Geometry: final body of the model. Coordinates: model frame, mm. A direction names the side the tool comes from. Give positions to 0.01 mm unless a question says otherwise; leave off trailing zeros. Loops run counter-clockwise (first coordinate to the right, second up) from the corner with the lowest first, then second, coordinate; pieces in that order, holes last.
from build123d import *

# Parameters (mm, degrees)
F0_W     = 1092.2
F0_H     = 744.5375
F0_W_2   = 920.75
F0_H_2   = 514.35
F1_DEPTH = 127
F2_W     = 1066.8
F2_H     = 25.4
F3_DEPTH = 25.4
F4_SIZE  = 9.525
F5_R     = 12.7
F6_DEPTH = 1066.8
F8_DEPTH = 6.35


with BuildPart() as f1:
    # F0 (on Top) → F1 (new body)
    with BuildSketch(Plane.XY):
        with Locations((546.1, 372.26875)):
            Rectangle(F0_W, F0_H)
        with Locations((527.05, 382.5875)):
            Rectangle(F0_W_2, F0_H_2, mode=Mode.SUBTRACT)
    extrude(amount=F1_DEPTH)

    # F2 (on face) → F3 (join)
    with BuildSketch(Plane.XY.offset(127)):
        with Locations((546.1, 31.75)):
            Rectangle(F2_W, F2_H)
        with Locations((546.1, 708.025)):
            Rectangle(F2_W, F2_H)
    extrude(amount=F3_DEPTH)

    # F4
    f4_edges = [f1.edges().sort_by_distance(p)[0] for p in [
        (546.1, 19.05, 152.4),
        (546.1, 44.45, 152.4),
        (546.1, 720.725, 152.4),
        (546.1, 695.325, 152.4),
    ]]
    chamfer(f4_edges, length=F4_SIZE)

    # F5 (on face) → F6 (join)
    with BuildSketch(Plane(origin=(12.7, 0, 0), x_dir=(0, -1, 0), z_dir=(-1, 0, 0))):
        with Locations((-708.025, 158.75)):
            Circle(F5_R)
        with BuildLine():
            Line((-34.925, 152.4), (-39.001326, 148.323674))
            ThreePointArc((-39.001326, 148.323674), (-31.75, 146.05), (-24.498674, 148.323674))
            Line((-24.498674, 148.323674), (-28.575, 152.4))
            Line((-28.575, 152.4), (-34.925, 152.4))
        make_face()
        with BuildLine():
            ThreePointArc((-24.498674, 148.323674), (-20.494294, 152.867902), (-19.05, 158.75))
            ThreePointArc((-19.05, 158.75), (-37.632098, 170.005706), (-39.001326, 148.323674))
            Line((-39.001326, 148.323674), (-34.925, 152.4))
            Line((-34.925, 152.4), (-28.575, 152.4))
            Line((-28.575, 152.4), (-24.498674, 148.323674))
        make_face()
    extrude(amount=-F6_DEPTH)

    # F7 (on face) → F8 (join)
    with BuildSketch(Plane.XY.offset(127)):
        Polygon((0, 0), (31.75, 0), (31.75, 19.05), (12.7, 19.05), (12.7, 44.45), (31.75, 44.45), (31.75, 133.35), (0, 133.35), align=None)
        Polygon((0, 744.5375), (0, 611.1875), (31.75, 611.1875), (31.75, 695.325), (12.7, 695.325), (12.7, 720.725), (31.75, 720.725), (31.75, 744.5375), align=None)
        Polygon((1060.45, 611.1875), (1092.2, 611.1875), (1092.2, 744.5375), (1060.45, 744.5375), (1060.45, 720.725), (1079.5, 720.725), (1079.5, 695.325), (1060.45, 695.325), align=None)
        Polygon((1060.45, 0), (1092.2, 0), (1092.2, 133.35), (1060.45, 133.35), (1060.45, 44.45), (1079.5, 44.45), (1079.5, 19.05), (1060.45, 19.05), align=None)
    extrude(amount=F8_DEPTH)


solid = f1.part
Item 1: Section query C-C on y = 560. Return loops of the section in (x, z) (3 decimals), plus the area to 3 significant figures.
Values follow:
outline: (0, 0) - (66.675, 0) - (66.675, 127) - (0, 127) - close; (987.425, 0) - (1092.2, 0) - (1092.2, 127) - (987.425, 127) - close
area: 21,800 mm2
Item 2: Set-up query: faces 1 (the face through (1079.5, 32, 152)), 2 (the face through (66.675, 379, 63)), 3 (the face through (12.7, 708, 153)). Return all of +Z, -Z, +X, -X, +Y, -Y with unobstructed straight access to the full face (end or side cutting, diameter ignored); none if empty.
Values follow:
face 1: +Z, +X, +Y, -Y
face 2: +Z, -Z
face 3: +Z, -X, +Y, -Y
Item 3: Section query A-A on z = 15.5. Return loops of the section in (x, y) (1 decimal).
Values follow:
outline: (0, 0) - (1092.2, 0) - (1092.2, 744.5) - (0, 744.5) - close; hole (66.7, 125.4) - (987.4, 125.4) - (987.4, 639.8) - (66.7, 639.8) - close
Item 4: Pin query (flat end, axial travel): pin 1 (8 mm diameter, centred on x = 785, z = 136, fed in from -Y); pin 2 (12.5 mm diameter, centred on y = 710, z = 158.5, fed in from -X); pin 3 (5 mm diameter, centred on x = 686.5, z = 138, fed in from +Y) (3 decimals). Return the tip coordinate at first contact, or that it passes through.
Values follow:
pin 1: stops at y = 19.05
pin 2: stops at x = 12.7
pin 3: stops at y = 720.725
Item 5: Ray query, probe 1 along Y at (x, z) = (414.5, 132) (3 decimals); probe 2 along X at (y, z) = (328.5, 57) (3 decimals); probe 3 along Y at (x, z) = (923, 117.5). Return the intervals inside material, ascending.
Values follow:
probe 1: y = 19.05 to 44.45, 695.325 to 720.725
probe 2: x = 0 to 66.675, 987.425 to 1092.2
probe 3: y = 0 to 125.41, 639.76 to 744.54
Item 6: Draft query along Z for faces 4 (the face through (538.63, 707.57, 171.44)), 5 (the face through (521, 639.762, 63)), 6 (the face through (538, 47, 0)). Return one class per face: +Z half, -Z half, draft (parallel to the pull), parting line (faces both ways), or undercut.
Values follow:
face 4: undercut
face 5: draft
face 6: -Z half
